Source: CAD feature listing. Evaluate the final solid. Frame: model axes, mm. Face numbers are marked on the shaded views. A direction names the side the tool comes from. Give positions to 0.01 mm unless a question says otherwise; leave off trailing zeros. Order: outer loops, then holes, each group sorted by start corner. A loop starts at its lowest first (then second) coordinate and runs counter-clockwise, first axis right, second up. Notation, with made-up numbers: M 31.5,8.5 L 77.5,8.5 A33 cw 77.5,40.5 Z; hole C 78.25,-39 d4. An arc over 180 degrees is marked long. Use CSV: the item, a comma, the result in double quotes. Start each with the question number.
Item 1: Section query A-A on x = 0. Return loops of the section in (y, z) (3 decimals).
Item 2: Section query B-B on z = 0. Return loops of the section in (x, y) (3 decimals).
Item 3: Access query for the marked faces 1, 2 and 3. Directions: +Z, -Z, +X, -X, +Y, -Y. A direction counts if a zero-diameter tool reaches every point of the face in a straight line with its end or side. Return the directions, or none.
Item 4: Section query C-C on y = -6. Return loops of the section in (x, z) (3 decimals).
Item 5: Section query D-D on z = 3.5. Return loops of the section in (x, y).
Item 6: Ray query, probe 1 along Y at (x, z) = (-2, -3); probe 2 along Y at (x, z) = (4.75, -1.5); probe 3 along Z at (x, y) = (0.25, 11). Return the intervals inside material, ascending. Write a range as from..to.
Item 7: First-contact query: pin 1 (1 mm diameter, centred on x = 1.5, y = 8, fed in from +Z); pin 2 (1 mm diameter, centred on x = -4, z = 4, fed in from +Y); pin 3 (1 mm diameter, centred on y = -5.5, z = 1, fed in from -X); pin 4 (1.5 mm diameter, centred on x = 4.5, y = -4.5, fed in from -Z). Flat tips, straight axial feed; report the tip coordinate or a pass-through.
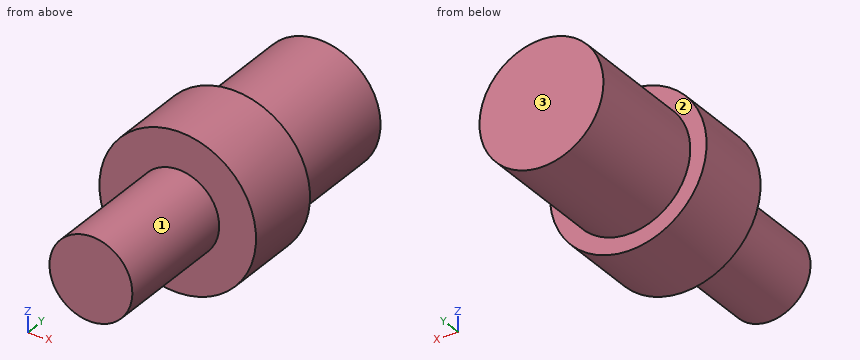
from build123d import *

# Parameters (mm, degrees)
SKETCH1_R           = 6
BOSS_EXTRUDE1_DEPTH = 3.11
SKETCH2_R           = 4.75
BOSS_EXTRUDE2_DEPTH = 10
SKETCH3_R           = 3.175
BOSS_EXTRUDE3_DEPTH = 10


with BuildPart() as part:
    # Sketch1 → Boss-Extrude1 (new, symmetric)
    with BuildSketch(Plane(origin=(0, 0, 0), x_dir=(1, 0, 0), z_dir=(0, 1, 0))):
        with Locations(Location((0, 0, 0), (0, 0, 270))):
            Circle(SKETCH1_R)
    extrude(amount=BOSS_EXTRUDE1_DEPTH, both=True)

    # Sketch2 → Boss-Extrude2 (add)
    with BuildSketch(Plane(origin=(0, 3.11, 0), x_dir=(1, 0, 0), z_dir=(0, 1, 0))):
        with Locations(Location((0, 0, 0), (0, 0, 270))):
            Circle(SKETCH2_R)
    extrude(amount=BOSS_EXTRUDE2_DEPTH)

    # Sketch3 → Boss-Extrude3 (add)
    with BuildSketch(Plane.XZ.offset(3.11)):
        with Locations(Location((0, 0, 0), (0, 0, 270))):
            Circle(SKETCH3_R)
    extrude(amount=BOSS_EXTRUDE3_DEPTH)


solid = part.part
Verdict:
1,outline,"M -13.11,-3.175 L -3.11,-3.175 L -3.11,-6 L 3.11,-6 L 3.11,-4.75 L 13.11,-4.75 L 13.11,4.75 L 3.11,4.75 L 3.11,6 L -3.11,6 L -3.11,3.175 L -13.11,3.175 Z"
2,outline,"M -6,-3.11 L -3.175,-3.11 L -3.175,-13.11 L 3.175,-13.11 L 3.175,-3.11 L 6,-3.11 L 6,3.11 L 4.75,3.11 L 4.75,13.11 L -4.75,13.11 L -4.75,3.11 L -6,3.11 Z"
3,face 1,"-Y"
3,face 2,"+Y"
3,face 3,"+Z, -Z, +X, -X, +Y"
4,outline,"C 0,0 d6.35"
5,outline,"M -4.87,-3.11 L 4.87,-3.11 L 4.87,3.11 L 3.21,3.11 L 3.21,13.11 L -3.21,13.11 L -3.21,3.11 L -4.87,3.11 Z"
6,probe 1,"-3.11..13.11"
6,probe 2,"-3.11..3.11"
6,probe 3,"-4.74..4.74"
7,pin 1,"z = 4.64"
7,pin 2,"y = 3.11"
7,pin 3,"x = -3.14"
7,pin 4,"through"
